Source: CAD feature listing. Evaluate the final solid. Frame: model axes, mm. Face numbers are marked on the shaded views. A direction names the side the tool comes from. Round coordinates to 2 decimals unless told otherwise and drop trailing zeros. Order: outer loops, then holes, each group sorted by start corner. A loop starts at its lowest first (then second) coordinate and runs counter-clockwise, first axis right, second up. Notation, with made-up numbers: (-31, -4) - (20, -4) arc R22 cw to (20, 30) - close; hole circle Ø3 at (49.5, 32.5). An arc over 180 degrees is marked (long way). Put each result on its own line as item: value. Start each with the question number.
1) Section C-C on y = -24. Output: boundary loops of the cut face in (x, z) (3 decimals).
2) Mould query, pull axis Z, two halves, no side actions, for the marked faces 1, 2 and 3. Classes: +Z half, -Z half, draft (parallel to the pull), parting line (faces both ways), or undercut.
3) Line query: probe 1 along Y at (x, z) = (-127, 210); probe 2 along Z at (x, y) = (-86, 371); probe 3 along X at (y, z) = (-219, -124) (3 decimals). Output: solid intervals per line, ascending. Write a range as [from, to].
4) Section B-B on x = 67. Output: boundary loops of the cut face in (y, z).
5) Access query for the marked faces 4 and 5. Directions: +Z, -Z, +X, -X, +Y, -Y. A direction counts if a zero-diameter tool reaches every point of the face in a straight line with its end or side. Return the directions, or none.
6) Section D-D on z = 74.5. Output: boundary loops of the cut face in (x, y) (3 decimals), then the cut area to 3 significant figures.
7) Contact query for flat-ended pins moving along their axis: P1, Ø16, axis at x = -127, y = -248.59, coming from the +Z side; P2, Ø12, axis at y = 390, z = -0.5, coming from the +X side (3 decimals). Output: stop coordinate, or through.
8) Section A-A on x = -127. Output: boundary loops of the cut face in (y, z), then the cut area to 3 significant figures.
```python
from build123d import *

# Parameters (mm, degrees)
F1_DEPTH = 508
F3_D     = 26.9875
F3_DEPTH = 25.4


with BuildPart() as f1:
    # F0 (on Front) → F1 (new body, symmetric)
    with BuildSketch(Plane.XZ):
        with BuildLine():
            Line((203.2, -228.6), (203.2, -203.2))
            Line((203.2, -203.2), (12.065, -203.2))
            ThreePointArc((12.065, -203.2), (10.268949, -202.456051), (9.525, -200.66))
            Line((9.525, -200.66), (9.525, 200.66))
            ThreePointArc((9.525, 200.66), (10.268949, 202.456051), (12.065, 203.2))
            Line((12.065, 203.2), (203.2, 203.2))
            Line((203.2, 203.2), (203.2, 228.6))
            Line((203.2, 228.6), (-203.2, 228.6))
            Line((-203.2, 228.6), (-203.2, 203.2))
            Line((-203.2, 203.2), (-12.065, 203.2))
            ThreePointArc((-12.065, 203.2), (-10.268949, 202.456051), (-9.525, 200.66))
            Line((-9.525, 200.66), (-9.525, -200.66))
            ThreePointArc((-9.525, -200.66), (-10.268949, -202.456051), (-12.065, -203.2))
            Line((-12.065, -203.2), (-203.2, -203.2))
            Line((-203.2, -203.2), (-203.2, -228.6))
            Line((-203.2, -228.6), (203.2, -228.6))
        make_face()
    extrude(amount=F1_DEPTH, both=True)

    # F3
    with Locations(Plane.XY.offset(228.6)):
        with Locations((-127, 183.212104), (-127, 56.212104), (-127, -248.587896), (127, -248.587896), (127, 56.212104), (127, 183.212104)):
            Hole(F3_D / 2, depth=F3_DEPTH)


solid = f1.part
```
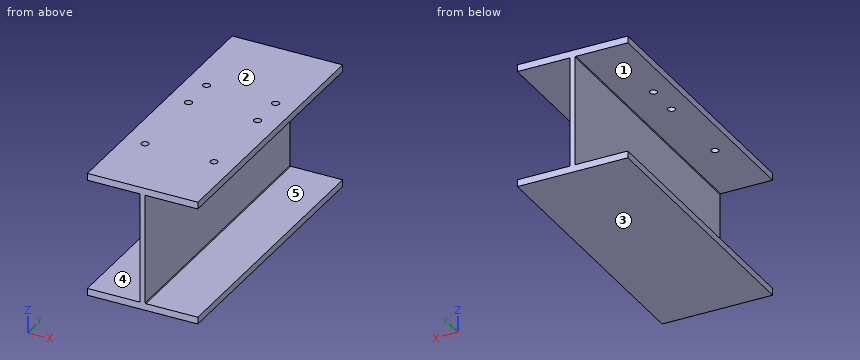
Answer sheet:
1. outline: (-203.2, -228.6) - (203.2, -228.6) - (203.2, -203.2) - (12.065, -203.2) arc R2.54 cw to (9.525, -200.66) - (9.525, 200.66) arc R2.54 cw to (12.065, 203.2) - (203.2, 203.2) - (203.2, 228.6) - (-203.2, 228.6) - (-203.2, 203.2) - (-12.065, 203.2) arc R2.54 cw to (-9.525, 200.66) - (-9.525, -200.66) arc R2.54 cw to (-12.065, -203.2) - (-203.2, -203.2) - close
2. face 1: undercut
2. face 2: +Z half
2. face 3: -Z half
3. probe 1: [-508, -262.08], [-235.09, 42.72], [69.71, 169.72], [196.71, 508]
3. probe 2: [-228.6, -203.2], [203.2, 228.6]
3. probe 3: [-9.525, 9.525]
4. outline: (-508, -228.6) - (508, -228.6) - (508, -203.2) - (-508, -203.2) - close; (-508, 203.2) - (508, 203.2) - (508, 228.6) - (-508, 228.6) - close
5. face 4: -X, +Y, -Y
5. face 5: +X, +Y, -Y
6. outline: (-9.525, -508) - (9.525, -508) - (9.525, 508) - (-9.525, 508) - close
6. area: 19,400 mm^2
7. P1: z = -203.2
7. P2: x = 9.525
8. outline: (-508, -228.6) - (508, -228.6) - (508, -203.2) - (-508, -203.2) - close; (-508, 203.2) - (-262.08, 203.2) - (-262.08, 228.6) - (-508, 228.6) - close; (-235.09, 203.2) - (42.72, 203.2) - (42.72, 228.6) - (-235.09, 228.6) - close; (69.71, 203.2) - (169.72, 203.2) - (169.72, 228.6) - (69.71, 228.6) - close; (196.71, 203.2) - (508, 203.2) - (508, 228.6) - (196.71, 228.6) - close
8. area: 49,600 mm^2
